from build123d import *

# Parameters (mm, degrees)
F0_R        = 5
F1_DEPTH    = 4
F2_W        = 10
F2_H        = 2
F2_W_2      = 18
F2_W_3      = 2
F2_H_2      = 14
F3_DEPTH    = 12
F4_R        = 5
F5_T1_DEPTH = 4
F6_R        = 1.5
F7_R        = 3.25
F9_DEPTH    = 2
F8_R        = 1.75
F10_DEPTH   = 2


# Not quite as in the source:
# - a fillet or chamfer that OpenCascade refuses, or shapes differently, is made with other operations: its cross-section is extruded or revolved along the edge and cut away or added


with BuildPart() as f1:
    # F0 (on Top) → F1 (new body)
    with BuildSketch(Plane.XY):
        Polygon((-24.0443362383, -18.3656413368), (31.299512524, 11.1093264446), (31.299512524, 13.1093264446), (36.7056637617, 13.1093264446), (36.7056637617, 15.1093264446), (-28.0443362383, 15.1093264446), (-28.0443362383, -34.8906735554), (-24.0443362383, -34.8906735554), align=None)
        Polygon((-24.0443362383, -13.8337272738), (-24.0443362383, 11.1093264446), (-11.0443362383, 11.1093264446), (3.6275881428, 11.1093264446), (22.7901370984, 11.1093264446), (3.6275881428, 0.9037566169), (-11.0443362383, -6.9102011778), align=None, mode=Mode.SUBTRACT)
        Polygon((3.6275881428, 11.1093264446), (-11.0443362383, 11.1093264446), (-11.0443362383, -6.9102011778), (3.6275881428, 0.9037566169), align=None)
        with Locations((-3.3724118572, 4.1093264446)):
            Circle(F0_R, mode=Mode.SUBTRACT)
    extrude(amount=F1_DEPTH)

    # F2 (on Top) → F3 (join)
    with BuildSketch(Plane.XY):
        with Locations((17.9556637617, 14.1093264446)):
            Rectangle(F2_W, F2_H)
        with Locations((-17.0443362383, 14.1093264446)):
            Rectangle(F2_W_2, F2_H)
        Polygon((-26.0443362383, 15.1093264446), (-28.0443362383, 15.1093264446), (-28.0443362383, -2.8906735554), (-26.0443362383, -2.8906735554), (-26.0443362383, 13.1093264446), align=None)
        with Locations((-27.0443362383, -27.8906735554)):
            Rectangle(F2_W_3, F2_H_2)
    extrude(amount=F3_DEPTH)

    # F4
    f4_edges = [f1.edges().sort_by_distance(p)[0] for p in [
        (-24.044336, 11.109326, 2),
        (-24.044336, -13.833727, 2),
        (-11.044336, -6.910201, 2),
        (-11.044336, 11.109326, 2),
        (-24.044336, -18.365641, 2),
        (-27.044336, -2.890674, 4),
        (-27.044336, -20.890674, 4),
        (-8.044336, 14.109326, 4),
        (12.955664, 14.109326, 4),
        (22.955664, 14.109326, 4),
    ]]
    fillet(f4_edges, radius=F4_R)

    # F5: fillet of radius 2.5 on 4 edges, made by hand

    # F5_s2 → F5_t1 (join)
    with BuildSketch(Plane.XY):
        with BuildLine():
            ThreePointArc((31.299512524, 11.1093264446), (32.1678634367, 12.5458181177), (33.7490022668, 13.1093264446))
            Line((33.7490022668, 13.1093264446), (31.299512524, 13.1093264446))
            Line((31.299512524, 13.1093264446), (31.299512524, 11.1093264446))
        make_face()
        with BuildLine():
            ThreePointArc((6.1275881428, 11.1093264446), (4.3598211899, 10.3770933976), (3.6275881428, 8.6093264446))
            Line((3.6275881428, 8.6093264446), (3.6275881428, 11.1093264446))
            Line((3.6275881428, 11.1093264446), (6.1275881428, 11.1093264446))
        make_face()
        with BuildLine():
            ThreePointArc((7.302762524, 2.8610770581), (4.840719065, 2.9242958576), (3.6275881428, 5.0676502325))
            Line((3.6275881428, 5.0676502325), (3.6275881428, 0.9037566169))
            Line((3.6275881428, 0.9037566169), (7.302762524, 2.8610770581))
        make_face()
        with BuildLine():
            ThreePointArc((12.7776375713, 11.1093264446), (15.2031718358, 9.2149530062), (13.9528119525, 6.4027532703))
            Line((13.9528119525, 6.4027532703), (22.7901370984, 11.1093264446))
            Line((22.7901370984, 11.1093264446), (12.7776375713, 11.1093264446))
        make_face()
    extrude(amount=F5_T1_DEPTH)

    # F6
    f6_edges = [f1.edges().sort_by_distance(p)[0] for p in [
        (-24.044336, -34.890674, 2),
    ]]
    fillet(f6_edges, radius=F6_R)

    # F7 (on face) → F9 (cut)
    with BuildSketch(Plane(origin=(0, 15.1093264446, 0), x_dir=(-1, 0, 0), z_dir=(0, 1, 0))):
        with Locations((-17.7056637617, 8)):
            Circle(F7_R)
        with Locations((13.0443362383, 8)):
            Circle(F7_R)
    extrude(amount=-F9_DEPTH, mode=Mode.SUBTRACT)

    # F8 (on face) → F10 (cut)
    with BuildSketch(Plane(origin=(-28.0443362383, 0, 0), x_dir=(0, -1, 0), z_dir=(-1, 0, 0))):
        with Locations((-2.1093264446, 8)):
            Circle(F8_R)
        with Locations((27.8906735554, 8)):
            Circle(F8_R)
    extrude(amount=-F10_DEPTH, mode=Mode.SUBTRACT)


solid = f1.part
Check sheet for the modelled part. Datum: model origin and axes. Units: mm. A direction names the side the tool comes from. Round coordinates to 2 decimals unless told otherwise and drop trailing zeros. Order: outer loops, then holes, each group sorted by start corner. A loop starts at its lowest first (then second) coordinate and runs counter-clockwise, first axis right, second up.
(1) Draft check along Z on faces 1 (the cylindrical face through (-27.06, -29.56, 8.53)), 2 (the flat face through (-8, 1, 0)), 3 (the flat face through (36.706, 14, 2)), 4 (the cylindrical face through (20.953, 14.123, 8.143)). Enter one of: pulls with the +Z half, pulls with the -Z half, needs draft (parallel to the pull), parting line crosses it, or undercut.
(2) Go/stop test with flat-tipped pins: P1, Ø4.5, axis at x = 8.5, z = 1.5, coming from the -Y side; P2, Ø6.5, axis at y = -21.5, z = 6.5, coming from the +X side; P3, Ø1.5, axis at x = 28.5, z = 4.5, coming from the -Y side. Record where each tip stops, or that it passes through.
(3) Scan lines: probe 1 along Y at (x, z) = (-17, 6.25); probe 2 along Y at (x, z) = (-1, 2.75); probe 3 along X at (y, z) = (4, 6). Record each from-to range of solid material in increasing order.
(4) Cross-section at C-C, the plane z = 8. State how many separate pieces and enclosed holes the cut face has, and give its area (3 significant figures).
(5) Cross-section at A-A, the plane y = -27. Enter the section's corners in (x, z), and give its area (3 significant figures).
(6) Cross-section at B-B, the plane x = -18. Enter the section's corners in (y, z).
(7) Access from +Z, -Z, +X, -X, +Y, -Y to the whole of each face (thin tool, end or side, straight path). Record for faces 5 (the flat face through (20, 13.109, 5)), 6 (the cylindrical face through (-27.06, -4.39, 5.43)), 7 (the flat face through (35, 13.109, 2)), 8 (the flat face through (-11.044, 1, 2)).
Check sheet entries:
1. face 1: undercut
1. face 2: pulls with the -Z half
1. face 3: needs draft
1. face 4: undercut
2. P1: stops at y = -2.23
2. P2: stops at x = -23.65
2. P3: stops at y = 9.32
3. probe 1: y = 13.11 to 15.11
3. probe 2: y = -6.09 to -0.29, 8.51 to 15.11
3. probe 3: x = -28.04 to -26.04
4. separate pieces: 7
4. enclosed holes: 0
4. area: 81.0 mm2
5. outline: (-28.04, 0) - (-24.04, 0) - (-24.04, 4) - (-26.04, 4) - (-26.04, 6.49) - (-28.04, 6.49) - close; (-28.04, 9.51) - (-26.04, 9.51) - (-26.04, 12) - (-28.04, 12) - close
5. area: 26.0 mm2
6. outline: (-15.15, 0) - (-10.4, 0) - (-10.4, 4) - (-15.15, 4) - close; (11.11, 0) - (15.11, 0) - (15.11, 12) - (13.11, 12) - (13.11, 4) - (11.11, 4) - close
7. face 5: +Z, +X, -Y
7. face 6: +Z, +X, -X
7. face 7: +Z, -Z, +X, -Y
7. face 8: +Z, -Z
